from build123d import *

# Parameters (mm, degrees)
F1_DEPTH = 21
F2_START = 19
F2_DEPTH = 2
F0_R     = 3.05
F3_DEPTH = 2


with BuildPart() as f1:
    # F0 (on Top) → F1 (new body)
    with BuildSketch(Plane.XY):
        Polygon((22.5, -9), (22.5, 0), (20.5, 0), (20.5, -7), (-20.5, -7), (-20.5, 0), (-22.5, 0), (-22.5, -9), align=None)
        Polygon((22.5, 0), (22.5, 9), (-22.5, 9), (-22.5, 0), (-20.5, 0), (-20.5, 7), (20.5, 7), (20.5, 0), align=None)
    extrude(amount=F1_DEPTH)

    # F0 (on Top) → F2 (join)
    with BuildSketch(Plane.XY.offset(F2_START)):
        with BuildLine():
            Line((16.1, 0), (20.5, 0))
            Line((20.5, 0), (20.5, 7))
            Line((20.5, 7), (-20.5, 7))
            Line((-20.5, 7), (-20.5, 0))
            Line((-20.5, 0), (-16.1, 0))
            ThreePointArc((-16.1, 0), (-13.5, 2.6), (-10.9, 0))
            Line((-10.9, 0), (-7.1, 0))
            ThreePointArc((-7.1, 0), (-4.5, 2.6), (-1.9, 0))
            Line((-1.9, 0), (1.9, 0))
            ThreePointArc((1.9, 0), (4.5, 2.6), (7.1, 0))
            Line((7.1, 0), (10.9, 0))
            ThreePointArc((10.9, 0), (13.5, 2.6), (16.1, 0))
        make_face()
        with BuildLine():
            Line((20.5, -7), (20.5, 0))
            Line((20.5, 0), (16.1, 0))
            ThreePointArc((16.1, 0), (13.5, -2.6), (10.9, 0))
            Line((10.9, 0), (7.1, 0))
            ThreePointArc((7.1, 0), (4.5, -2.6), (1.9, 0))
            Line((1.9, 0), (-1.9, 0))
            ThreePointArc((-1.9, 0), (-4.5, -2.6), (-7.1, 0))
            Line((-7.1, 0), (-10.9, 0))
            ThreePointArc((-10.9, 0), (-13.5, -2.6), (-16.1, 0))
            Line((-16.1, 0), (-20.5, 0))
            Line((-20.5, 0), (-20.5, -7))
            Line((-20.5, -7), (20.5, -7))
        make_face()
    extrude(amount=F2_DEPTH)

    # F0 (on Top) → F3 (join)
    with BuildSketch(Plane.XY):
        Polygon((-32.5, 19), (-32.5, 14), (-32.5, -19), (32.5, -19), (32.5, 19), align=None)
        with BuildLine():
            ThreePointArc((-24.45, 14), (-25.3433243174, 11.8433243174), (-27.5, 10.95))
            ThreePointArc((-27.5, 10.95), (-29.6566756826, 11.8433243174), (-30.55, 14))
            ThreePointArc((-30.55, 14), (-27.5, 17.05), (-24.45, 14))
        make_face(mode=Mode.SUBTRACT)
        Polygon((-22.5, 9), (22.5, 9), (22.5, 0), (22.5, -9), (-22.5, -9), (-22.5, 0), align=None, mode=Mode.SUBTRACT)
        with Locations((27.5, 14)):
            Circle(F0_R, mode=Mode.SUBTRACT)
    extrude(amount=F3_DEPTH)


solid = f1.part
Model file for the job. Use its own axes, mm. A direction names the side the tool comes from. Coordinates: 2 decimals unless noted, no trailing zeros. Write each loop counter-clockwise with the first axis right and the second up, starting at its lowest first coordinate (ties: lowest second). Pieces come first, ordered by that corner, then holes. Notation, with made-up numbers: (81.25, -15) - (111.25, -15) arc R9 ccw to (111.25, -9) - close; hole circle Ø1 at (-4, 71.5). An arc over 180 degrees is marked (long way). Write each question's results on one line, items separated by ' | '. Start each with the question number.
1) Flat gauge pins, fed straight in: P1, Ø5.5, axis at x = -3, z = 6.5, coming from the -Y side; P2, Ø8, axis at y = -4, z = 4, coming from the +X side; P3, Ø6, axis at x = -4.5, y = 0, coming from the -Z side; P4, Ø1.5, axis at y = -1.5, z = 16.5, coming from the -X side. Where does each tip first touch, or does it go through?
2) Cut at A-A (y = 0). Write the cut outline in (x, z).
3) Probe line 1 along Y through (x, z) = (4.5, 19.8); line 2 along X through (y, z) = (-2.5, 5.25); line 3 along Y through (x, z) = (-19, 6.5). List the from-to ranges inside material, lowest first. Write a range as from..to.
4) Cut at B-B (x = -13.5). Write the cut outline in (y, z), then the cut area to 3 significant figures.
5) Mould opens along Y. For faces 6 (the face through (30.41, 14.92, 0.99)), 7 (the face through (0, -9, 11)), 8 (the face through (-32.5, 0, 1)) say: pulls with the +Y half, pulls with the -Y half, needs draft (parallel to the pull), parting line crosses it, or undercut.
6) Cut at C-C (z = 8). Write the cut outline in (x, y).
7) 3-axis set-ups, long thin cutter, end or side, ignore diameter. For faces 1 (the face through (22.5, 0, 11)), 2 (the face through (0, -19, 1)), 3 (the face through (-20.5, 0, 9)), 4 (the face through (-11.02, -0.78, 19.99)), 5 (the face through (-22.5, 0, 11)): which of +Z, -Z, +X, -X, +Y, -Y reach the whole face in a straight line?
8) Cut at D-D (y = 13). Write the cut outline in (x, z).
Returned:
1) P1: y = -9 | P2: x = 32.5 | P3: z = 19 | P4: x = -22.5
2) outline: (-32.5, 0) - (-20.5, 0) - (-20.5, 19) - (-16.1, 19) - (-16.1, 21) - (-22.5, 21) - (-22.5, 2) - (-32.5, 2) - close; (-10.9, 19) - (-7.1, 19) - (-7.1, 21) - (-10.9, 21) - close; (-1.9, 19) - (1.9, 19) - (1.9, 21) - (-1.9, 21) - close; (7.1, 19) - (10.9, 19) - (10.9, 21) - (7.1, 21) - close; (16.1, 19) - (20.5, 19) - (20.5, 0) - (32.5, 0) - (32.5, 2) - (22.5, 2) - (22.5, 21) - (16.1, 21) - close
3) line 1: -9..-2.6, 2.6..9 | line 2: -22.5..-20.5, 20.5..22.5 | line 3: -9..-7, 7..9
4) outline: (-19, 0) - (-7, 0) - (-7, 19) - (-2.6, 19) - (-2.6, 21) - (-9, 21) - (-9, 2) - (-19, 2) - close; (2.6, 19) - (7, 19) - (7, 0) - (19, 0) - (19, 2) - (9, 2) - (9, 21) - (2.6, 21) - close | area: 142 mm^2
5) face 6: undercut | face 7: pulls with the -Y half | face 8: needs draft
6) outline: (-22.5, -9) - (22.5, -9) - (22.5, 9) - (-22.5, 9) - close; hole (-20.5, -7) - (20.5, -7) - (20.5, 7) - (-20.5, 7) - close
7) face 1: +Z, +X, +Y, -Y | face 2: +Z, -Z, +X, -X, -Y | face 3: -Z | face 4: +Z, -Z | face 5: +Z, -X, +Y, -Y
8) outline: (-32.5, 0) - (-30.38, 0) - (-30.38, 2) - (-32.5, 2) - close; (-24.62, 0) - (24.62, 0) - (24.62, 2) - (-24.62, 2) - close; (30.38, 0) - (32.5, 0) - (32.5, 2) - (30.38, 2) - close
